```python
from build123d import *

# Parameters (mm, degrees)
SKETCH1_R           = 3
BOSS_EXTRUDE1_DEPTH = 5
SKETCH2_R           = 3
BOSS_EXTRUDE2_DEPTH = 15


with BuildPart() as part:
    # Sketch1 → Boss-Extrude1 (new body)
    with BuildSketch(Plane.XY):
        Polygon((-12.258432753, 2.072266385), (38.505942563, 14.841548426), (54.906660914, -36.079753149), align=None)
        Circle(SKETCH1_R, mode=Mode.SUBTRACT)
        with Locations((35.591293936, 8.952641841)):
            Circle(SKETCH1_R, mode=Mode.SUBTRACT)
    extrude(amount=BOSS_EXTRUDE1_DEPTH)

    # Sketch2 → Boss-Extrude2 (add)
    with BuildSketch(Plane(origin=(0, 0, 0), x_dir=(-1, 0, 0), z_dir=(0, 0, -1))):
        with Locations((-35.591293936, 8.952641841)):
            Circle(SKETCH2_R)
    extrude(amount=-BOSS_EXTRUDE2_DEPTH)


solid = part.part
```
Verification items for the finished model (mm, model axes). Round coordinates to 2 decimals unless told otherwise and drop trailing zeros. Loops run counter-clockwise (first coordinate to the right, second up) from the corner with the lowest first, then second, coordinate; pieces in that order, holes last. Notation, with made-up numbers: (53.25, 54.25) -> (79.25, 54.25) arc R20 cw to (79.25, 84.25) -> close; hole circle Ø1 at (-30, -8.5). An arc over 180 degrees is marked (long way). Answer as a JSON object with one key per item and string values.
Q1. Go/stop test with flat-tipped pins: P1, Ø2, axis at x = 33.5, z = 12, coming from the +Y side; P2, Ø5, axis at y = -13, z = 4.5, coming from the -X side; P3, Ø6, axis at x = 38, y = -23.5, coming from the +Z side. Record where each tip stops, or that it passes through.
Data:
{"P1": "stops at y = 11.75", "P2": "stops at x = 9.87", "P3": "stops at z = 5"}
Q2. Section check B-B (x = 0). Record the boundary of the cut face in (y, z).
Data:
{"outline": "(-4.89, 0) -> (-3, 0) -> (-3, 5) -> (-4.89, 5) -> close; (3, 0) -> (5.16, 0) -> (5.16, 5) -> (3, 5) -> close"}
Q3. Draft check along X on faces 1 (the flat face through (29, -5, 0)), 2 (the cylindrical face through (32.73, 9.85, 9.93)), 3 (the cylindrical face through (-3, 0, 2)), 4 (the flat face through (12.768, 8.368, 2.465)). Enter one of: pulls with the +X half, pulls with the -X half, needs draft (parallel to the pull), parting line crosses it, or undercut.
Data:
{"face 1": "needs draft", "face 2": "parting line crosses it", "face 3": "undercut", "face 4": "pulls with the -X half"}
Q4. Scan lines: line 1 (Y direction, x = 0, z = 3.05); line 2 (Z direction, x = 42, y = -28); line 3 (X direction, y = -7.5, z = 4.5). Record each from-to range of solid material in increasing order. Write a range as from..to.
Data:
{"line 1": "y = -4.89..-3, 3..5.16", "line 2": "z = 0..5", "line 3": "x = 4.59..45.7"}
Q5. Section check A-A (y = 0). Record the boundary of the cut face in (x, z), then the cut area to 3 significant figures.
Data:
{"outline": "(-8.61, 0) -> (-3, 0) -> (-3, 5) -> (-8.61, 5) -> close; (3, 0) -> (43.29, 0) -> (43.29, 5) -> (3, 5) -> close", "area": "229 mm2"}
Q6. Section check D-D (z = 6.5). Record the boundary of the cut face in (x, y).
Data:
{"outline": "circle Ø6 at (35.59, 8.95)"}
Q7. Section check C-C (z = 1.75). Record the boundary of the cut face in (x, y).
Data:
{"outline": "(-12.26, 2.07) -> (54.91, -36.08) -> (38.51, 14.84) -> close; hole circle Ø6 at (0, 0)"}
